Geometry check sheet. Reference: the model listing, model coordinates, mm. A direction names the side the tool comes from. Coordinates: 2 decimals unless noted, no trailing zeros. Order: outer loops, then holes, each group sorted by start corner. A loop starts at its lowest first (then second) coordinate and runs counter-clockwise, first axis right, second up. Notation, with made-up numbers: M -0.75,-9 L 56.25,-9 A25 cw 56.25,28 Z; hole C 80,0 d2. An arc over 180 degrees is marked long. Use CSV: the item, a comma, the result in double quotes. Start each with the question number.
Autodesk Inventor part; units mm, degrees
ref_plane "YZ Plane" through (0, 0, 0) normal (1, 0, 0) x (0, 1, 0)
ref_plane "XZ Plane" through (0, 0, 0) normal (0, 1, 0) x (-1, 0, 0)
ref_plane "XY Plane" through (0, 0, 0) normal (0, 0, 1) x (1, 0, 0)
sketch "Sketch1" plane through (0, 0, 0) normal (0, 1, 0) x (-1, 0, 0)
  line L0 (9, -16) -> (-9, -16)
  line L1 (-9, -16) -> (-9, 16)
  line L2 (-9, 16) -> (9, 16)
  line L3 (9, 16) -> (9, -16)
  line L4 (9, -16) -> (-9, 16) construction
  line L5 (-9, -16) -> (9, 16) construction
  circle A0 centre (0, 6.5) radius 4.8
  line L6 (0, 6.5) -> (0, -6.5)
  circle A1 centre (0, -6.5) radius 4.8
  line L7 (0, 11.3) -> (-9, 11.3)
  line L8 (0, 1.7) -> (-9, 1.7)
  line L9 (0, -1.7) -> (-9, -1.7)
  line L10 (0, -11.3) -> (-9, -11.3)
  point P0 (0, 0)
  point P1 (0, 0)
  dimension "d0" = 18
  dimension "d1" = 32
  dimension "d2" = 9.6
  dimension "d3" = 13
  dimension "d4" = 9.6
extrude "Extrusion1" add sketch "Sketch1" along normal blind 2 contours L0 L1 L10 A1 L6 A0 L7 L2 L3 | L1 L8 L6 L9
sketch "Sketch2" plane through (0, 0, 0) normal (0, -1, 0) x (1, 0, 0)
  line L0 (-9, 16) -> (9, 16)
  line L1 (9, 16) -> (-9, 16)
  line L2 (-9, -16) -> (-9, 16)
  line L3 (-9, 16) -> (-9, -16)
  line L4 (9, -16) -> (-9, -16)
  line L5 (-9, -16) -> (9, -16)
  line L6 (9, -16) -> (9, -14)
  line L7 (9, -11.3) -> (9, -16)
  line L8 (9, -14) -> (-7, -14)
  line L9 (-7, -14) -> (-7, 14)
  line L10 (-7, 14) -> (9, 14)
  line L11 (9, 16) -> (9, 11.3)
  point P0 (0, 0)
  dimension "d7" = 2
  dimension "d8" = 16
  dimension "d9" = 28
extrude "Extrusion2" add sketch "Sketch2" along normal blind 2.5
sketch "Sketch3" plane through (-9, 2, -16) normal (-1, 0, 0) x (0, 0, 1)
  line L0 (0, 0) -> (0, -4.5)
  line L1 (0, -4.5) -> (32, -4.5)
  line L2 (32, -4.5) -> (32, 50)
  line L3 (32, 50) -> (0, 50)
  line L4 (0, 50) -> (0, -4.5)
  point P0 (16, -2)
  dimension "d12" = 54.5
extrude "Extrusion3" add sketch "Sketch3" along normal blind 2
sketch "Sketch4" plane through (0, -2.5, 0) normal (0, -1, 0) x (1, 0, 0)
  line L0 (9, 16) -> (9, 11.3)
  line L1 (9, 16) -> (-36, 16)
  line L2 (-36, 16) -> (-36, -16)
  line L3 (-36, -16) -> (9, -16)
  line L4 (9, -16) -> (9, 16)
  point P0 (0, 0)
  dimension "d15" = 45
extrude "Extrusion4" add sketch "Sketch4" along normal blind 2
sketch "Sketch5" plane through (-7, 0, 14) normal (1, 0, 0) x (0, 0, -1)
  line L0 (0, 0) -> (0, -2.5)
  line L1 (30, -2.5) -> (-2, -2.5)
  line L2 (0, 0) -> (3, 0)
  line L3 (3, 0) -> (3, -2.5)
  line L4 (3, -2.5) -> (0, -2.5)
  line L5 (0, -2.5) -> (0, 0)
  point P0 (14, 0)
  dimension "d18" = 3
extrude "Extrusion5" cut sketch "Sketch5" against normal up to surface (4 mm away)
sketch "Sketch6" plane through (9, 0, 1.7) normal (1, 0, 0) x (0, 0, -1)
  line L0 (0, 0) -> (0, 2)
  line L1 (3.4, 0) -> (3.4, 2)
  line L2 (0, 1) -> (3.4, 1)
  line L3 (3.4, 1) -> (3.4, 2)
  line L4 (3.4, 2) -> (0, 2)
  line L5 (0, 2) -> (0, 1)
  point P0 (1.7, 0)
extrude "Extrusion6" cut sketch "Sketch6" against normal blind 2.2
sketch "Sketch8" plane through (-11, 2, -16) normal (-1, 0, 0) x (0, 0, 1)
  circle A0 centre (24.6, 39.75) radius 2.75
  circle A1 centre (24.6, 39.75) radius 1.4
  line L0 (4, 47.25) -> (28, 47.25) construction
  line L1 (28, 47.25) -> (28, -1.75) construction
  line L2 (28, -1.75) -> (4, -1.75) construction
  line L3 (4, -1.75) -> (4, 47.25) construction
  circle A2 centre (7.4, 5.75) radius 2.75
  circle A3 centre (7.4, 5.75) radius 1.4
  line L4 (4, 47.25) -> (28, -1.75) construction
  line L5 (32, -4.5) -> (32, -6.5) construction
  line L6 (32, 50) -> (0, 50) construction
  line L7 (0, -4.5) -> (32, 50) construction
  point P0 (16, -2)
  point P1 (16, 22.75)
  point P2 (16, 22.75)
  dimension "d24" = 5.5
  dimension "d25" = 2.8
  dimension "d26" = 24
  dimension "d27" = 49
  dimension "d28" = 3.4
  dimension "d29" = 7.5
  dimension "d30" = 5.5
  dimension "d31" = 2.8
  dimension "d32" = 3.4
  dimension "d33" = 7.5
extrude "Extrusion7" add sketch "Sketch8" along normal blind 5
properties part number "prototype7_1"
1) Set-up check for faces 5 (the face through (4, 1, -1.7)), 6 (the face through (-1, -1, 14)), 7 (the face through (-14, -2.5, 0)), 8 (the face through (-13.46, 8.6, -9.71)), 9 (the face through (-7, -1, -2)): record each of +Z, -Z, +X, -X, +Y, -Y from which the full face is reachable in a straight line by a thin tool's end or side.
2) Section check A-A on z = 12. Record the boundary of the cut face in (x, y).
3) Section check B-B on x = 4.5. Record the boundary of the cut face in (y, z).
4) Section check D-D on z = 1. Record the boundary of the cut face in (x, y), then the cut area to 3 significant figures.
5) Draft check along Z on faces 1 (the face through (-10, 7, 16)), 2 (the face through (-4.8, 1, 6.6)), 3 (the face through (-9, 27, 0)), 4 (the face through (-13.46, 40.36, 8.42)). Enter one of: +Z half, -Z half, draft (parallel to the pull), parting line (faces both ways), or undercut.
6) Gauge pin test, flat ends, axial feed: P1, Ø1, axis at y = 27, z = -3.5, coming from the +X side; P2, Ø5.5, axis at x = -3.5, z = 5, coming from the +Y side; P3, Ø1.2, axis at y = -1.5, z = -3, coming from the +X side. Record the tip position at first contact, or that the pin passes through.
7) Section check C-C on y = 41.75. Record the boundary of the cut face in (x, z), then the cut area to 3 significant figures.
8) Material ranges on line 1 along Y through (x, z) = (-13.95, 8.6); line 2 along Y through (x, z) = (-13.8, -8.6); line 3 along Y through (x, z) = (-5, -10.5), recorded low to high.
Results are:
1,face 5,"+X, +Y"
1,face 6,"+X, -X"
1,face 7,"none"
1,face 8,"-X"
1,face 9,"+X"
2,outline,"M -36,-4.5 L 9,-4.5 L 9,-2.5 L -36,-2.5 Z; M -11,0 L 9,0 L 9,2 L -9,2 L -9,52 L -11,52 Z"
3,outline,"M -4.5,-16 L 2,-16 L 2,-11.3 L 0,-11.3 L 0,-14 L -2.5,-14 L -2.5,14 L 0,14 L 0,11.3 L 2,11.3 L 2,16 L -4.5,16 Z; M 0,-1.7 L 2,-1.7 L 2,1.7 L 0,1.7 Z"
4,outline,"M -36,-4.5 L 9,-4.5 L 9,-2.5 L -7,-2.5 L -7,0 L 9,0 L 9,1 L 6.8,1 L 6.8,2 L -9,2 L -9,52 L -11,52 L -11,-2.5 L -36,-2.5 Z"
4,area,"238 mm²"
5,face 1,"+Z half"
5,face 2,"undercut"
5,face 3,"draft"
5,face 4,"undercut"
6,P1,"stops at x = -9"
6,P2,"stops at y = 2"
6,P3,"stops at x = -7"
7,outline,"M -16,5.85 L -11,5.85 L -11,-16 L -9,-16 L -9,16 L -11,16 L -11,11.35 L -16,11.35 L -16,10 L -11,10 L -11,7.2 L -16,7.2 Z"
7,area,"77.5 mm²"
8,line 1,"y = -4.5 to -2.5, 39 to 40.35, 43.15 to 44.5"
8,line 2,"y = -4.5 to -2.5, 5 to 6.35, 9.15 to 10.5"
8,line 3,"y = -4.5 to -2.5, 0 to 2"
